The listing builds one solid part. Answer for the finished solid, in the listing's coordinates (mm). Face numbers are marked on the shaded views. A direction names the side the tool comes from. Coordinates: 2 decimals unless noted, no trailing zeros. Loops run counter-clockwise (first coordinate to the right, second up) from the corner with the lowest first, then second, coordinate; pieces in that order, holes last. Notation, with made-up numbers: M 51,-18 L 56,-18 A5 ccw 56,-9 Z; hole C 33.25,34 d9. An arc over 180 degrees is marked long. Answer as a JSON object with one key per item and string values. Group by question number.
1. Straight lines are drawn through the part: L1, parallel to Y at x = 3, z = -16.5; L2, parallel to Z at x = 34.5, y = 13.5; L3, parallel to Z at x = 26, y = 11. For each, find the intervals that lie inside material, in ascending order.
2. For the marked faces 1, 2 and 3, determine the directions among +Z, -Z, +X, -X, +Y, -Y from which every point of the face is accessible in a straight line to the end or side of a thin tool.
3. A cutting plane is placed at A-A on y = 21.5. Give the vertices of the cut face in (x, z), and give its area (3 significant figures).
4. Given pin 1 (12 mm diameter, centred on y = 22.5, z = 20, fed in from +X); pin 2 (8 mm diameter, centred on x = 46, y = 24.5, fed in from +Z); pin 3 (5 mm diameter, centred on x = 29.5, y = 7, fed in from +Z), each flat-ended and moving along its own axis, determine where each tip first touches the part or whether it passes through.
5. A cutting plane is placed at B-B on y = 5. Give the vertices of the cut face in (x, z).
6. A cutting plane is placed at C-C on z = -16. Give the vertices of the cut face in (x, y), and give its area (3 significant figures).
7. Determine the mould class of the marked faces 4, 5, 6 and 7 for opening direction X: released by +X, released by -X, zero draft, split by the parting line, or undercut.
from build123d import *

# Parameters (mm, degrees)
P_IDAT_VYSUNUT_M2_DEPTH  = 30
ODEBRAT_VYSUNUT_M1_DEPTH = 30
ODEBRAT_VYSUNUT_M2_DEPTH = 30
ODEBRAT_VYSUNUT_M3_DEPTH = 30
ODEBRAT_VYSUNUT_M4_DEPTH = 30
ODEBRAT_VYSUNUT_M5_DEPTH = 24


with BuildPart() as part:
    # Skica2 → Přidat vysunutím2 (new body)
    with BuildSketch(Plane(origin=(0, 0, 0), x_dir=(1, 0, 0), z_dir=(0, 1, 0))):
        with BuildLine():
            Line((-68.909987848, 61.819805153), (-33.554648789, 26.464466094))
            ThreePointArc((-33.554648789, 26.464466094), (-30.731632254, 13.372688112), (-30, 0))
            ThreePointArc((-30, 0), (-30.722175449, -13.37191938), (-33.535533906, -26.464466094))
            Line((-33.535533906, -26.464466094), (-68.890872965, -61.819805153))
            Line((-68.890872965, -61.819805153), (-61.819805153, -68.890872965))
            Line((-61.819805153, -68.890872965), (-26.464466094, -33.535533906))
            ThreePointArc((-26.464466094, -33.535533906), (-13.37191938, -30.722175449), (0, -30))
            ThreePointArc((0, -30), (13.37191938, -30.722175449), (26.464466094, -33.535533906))
            Line((26.464466094, -33.535533906), (61.819805153, -68.890872965))
            Line((61.819805153, -68.890872965), (68.890872965, -61.819805153))
            Line((68.890872965, -61.819805153), (33.535533906, -26.464466094))
            ThreePointArc((33.535533906, -26.464466094), (30.722175449, -13.37191938), (30, 0))
            ThreePointArc((30, 0), (30.722175449, 13.37191938), (33.535533906, 26.464466094))
            Line((33.535533906, 26.464466094), (68.890872965, 61.819805153))
            Line((68.890872965, 61.819805153), (61.819805153, 68.890872965))
            Line((61.819805153, 68.890872965), (26.464466094, 33.535533906))
            ThreePointArc((26.464466094, 33.535533906), (13.37191938, 30.722175449), (0, 30))
            ThreePointArc((0, 30), (-13.381577193, 30.72066838), (-26.483580977, 33.535533906))
            Line((-26.483580977, 33.535533906), (-61.838920037, 68.890872965))
            Line((-61.838920037, 68.890872965), (-68.909987848, 61.819805153))
        make_face()
    extrude(amount=P_IDAT_VYSUNUT_M2_DEPTH)

    # Skica4 → Odebrat vysunutím1 (cut)
    with BuildSketch(Plane(origin=(3.535533906, 0, -3.535533906), x_dir=(-0.707106781186553, 0, -0.7071067811865421), z_dir=(0.7071067811865421, 0, -0.707106781186553))):
        with BuildLine():
            Line((-42.426406871, 0), (-92.426406871, 0))
            Line((-92.426406871, 0), (-92.426406871, 24))
            ThreePointArc((-92.426406871, 24), (-65.126443653, 16.791590037), (-42.426406871, 0))
        make_face()
    extrude(amount=-ODEBRAT_VYSUNUT_M1_DEPTH, mode=Mode.SUBTRACT)

    # Skica5 → Odebrat vysunutím2 (cut)
    with BuildSketch(Plane(origin=(3.535533906, 0, 3.535533906), x_dir=(0.7071067811865475, 0, -0.7071067811865477), z_dir=(0.7071067811865477, 0, 0.7071067811865475))):
        with BuildLine():
            Line((-92.426406871, 0), (-92.426406871, 24))
            ThreePointArc((-92.426406871, 24), (-65.126443653, 16.791590037), (-42.426406871, 0))
            Line((-42.426406871, 0), (-92.426406871, 0))
        make_face()
    extrude(amount=-ODEBRAT_VYSUNUT_M2_DEPTH, mode=Mode.SUBTRACT)

    # Skica6 → Odebrat vysunutím3 (cut)
    with BuildSketch(Plane(origin=(-3.545091348, 0, 3.545091348), x_dir=(0.7071067811865475, 0, 0.7071067811865476), z_dir=(-0.7071067811865476, 0, 0.7071067811865475))):
        with BuildLine():
            Line((-92.439923135, 0), (-92.439923135, 24))
            ThreePointArc((-92.439923135, 24), (-65.139959917, 16.791590037), (-42.439923135, 0))
            Line((-42.439923135, 0), (-92.439923135, 0))
        make_face()
    extrude(amount=-ODEBRAT_VYSUNUT_M3_DEPTH, mode=Mode.SUBTRACT)

    # Skica7 → Odebrat vysunutím4 (cut)
    with BuildSketch(Plane(origin=(-3.535533906, 0, -3.535533906), x_dir=(-0.7071067811865472, 0, 0.7071067811865478), z_dir=(-0.7071067811865478, 0, -0.7071067811865472))):
        with BuildLine():
            Line((-92.426406871, 0), (-92.426406871, 24))
            ThreePointArc((-92.426406871, 24), (-65.126443653, 16.791590037), (-42.426406871, 0))
            Line((-42.426406871, 0), (-92.426406871, 0))
        make_face()
    extrude(amount=-ODEBRAT_VYSUNUT_M4_DEPTH, mode=Mode.SUBTRACT)

    # Skica8 → Odebrat vysunutím5 (cut)
    with BuildSketch(Plane.XZ):
        with BuildLine():
            Line((-33.554648789, -26.464466094), (-33.535533906, 26.464466094))
            ThreePointArc((-33.535533906, 26.464466094), (-24.490727529, 24.490727529), (-26.464466094, 33.535533906))
            Line((-26.464466094, 33.535533906), (26.464466094, 33.535533906))
            ThreePointArc((26.464466094, 33.535533906), (24.490727529, 24.490727529), (33.535533906, 26.464466094))
            Line((33.535533906, 26.464466094), (33.535533906, -26.464466094))
            ThreePointArc((33.535533906, -26.464466094), (24.490727529, -24.490727529), (26.464466094, -33.535533906))
            Line((26.464466094, -33.535533906), (-26.483580977, -33.535533906))
            ThreePointArc((-26.483580977, -33.535533906), (-24.509842412, -24.490727529), (-33.554648789, -26.464466094))
        make_face()
    extrude(amount=-ODEBRAT_VYSUNUT_M5_DEPTH, mode=Mode.SUBTRACT)


solid = part.part
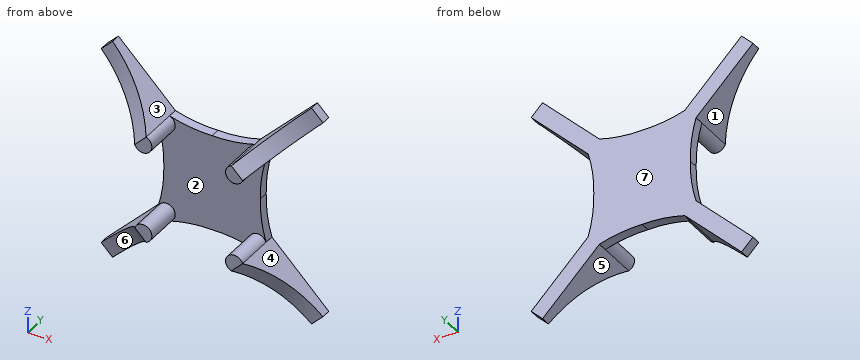
From the geometry:
{
 "1": {"L1": "y = 24 to 30", "L2": "z = -41.57 to -27.43, 27.43 to 41.57", "L3": "z = -33.34 to -23.42, 23.42 to 33.34"},
 "2": {"face 1": "-X, +Y, -Y", "face 2": "-Y", "face 3": "+Z, +Y, -Y"},
 "3": {"outline": "M -58.51,-51.42 L -51.44,-58.49 L -26.48,-33.54 A5.5 ccw long -33.55,-26.46 Z; M -58.49,51.42 L -33.54,26.46 A5.5 ccw long -26.46,33.54 L -51.42,58.49 Z; M 26.46,-33.54 L 51.42,-58.49 L 58.49,-51.42 L 33.54,-26.46 A5.5 ccw long Z; M 26.46,33.54 A5.5 ccw long 33.54,26.46 L 58.49,51.42 L 51.42,58.49 Z", "area": "1,700 mm²"},
 "4": {"pin 1": "stops at x = 33.34", "pin 2": "stops at z = 57.07", "pin 3": "stops at z = 39.05"},
 "5": {"outline": "M -37.14,-30.05 L -30.07,-37.12 L -26.48,-33.54 A5.5 ccw long -33.55,-26.46 Z; M -37.12,30.05 L -33.54,26.46 A5.5 ccw long -26.46,33.54 L -30.05,37.12 Z; M 26.46,-33.54 L 30.05,-37.12 L 37.12,-30.05 L 33.54,-26.46 A5.5 ccw long Z; M 26.46,33.54 A5.5 ccw long 33.54,26.46 L 37.12,30.05 L 30.05,37.12 Z"},
 "6": {"outline": "M -31.13,24 L 31.12,24 L 31.12,30 L -31.13,30 Z", "area": "373 mm²"},
 "7": {"face 4": "released by +X", "face 5": "undercut", "face 6": "released by -X", "face 7": "zero draft"}
}
